Part model, mm, in its own coordinate system. Face numbers are marked on the shaded views. A direction names the side the tool comes from. Round coordinates to 2 decimals unless told otherwise and drop trailing zeros. Loops run counter-clockwise (first coordinate to the right, second up) from the corner with the lowest first, then second, coordinate; pieces in that order, holes last. Notation, with made-up numbers: M 32,30.25 L 79,30.25 A9 cw 79,42.25 Z; hole C -20,4.5 d7. An arc over 180 degrees is marked long. Answer as CSV lines item,"result". Start each with the question number.
Item 1: Drop flat-ended pins along their axis: pin 1 Ø4 at (x, y) = (-15.875, -15.875) entering from -Z; pin 2 Ø2.5 at (x, z) = (0.5, 1.5) entering from -Y; pin 3 Ø1 at (x, y) = (12.5, -40.5) entering from +Z. Give the stop position or say it passes through.
Item 2: Wall check: line 1 (Y direction, x = 0, z = 2.75); line 2 (Z direction, x = -20.25, y = -53); line 3 (Y direction, x = -7.5, z = 3.5). Give the ranges that are in metal, low to high.
Item 3: Band-saw the part on B-B (y = -53). Give the cut face in (x, z).
Item 4: Band-saw the part on D-D (z = 8.5). Give the cut face in (x, y), and give its area (3 significant figures).
Item 5: Band-saw the part on C-C (x = 0). Give the cut face in (y, z).
Item 6: Mould opens along X. For the marked faces 4, 5, 6 and 7 say: pulls with the +X half, pulls with the -X half, needs draft (parallel to the pull), parting line crosses it, or undercut.
Item 7: Which spindle directions (+Z, -Z, +X, -X, +Y, -Y) get a long thin tool onto all of the face, cutting with end or side? Do the marked faces 1, 2 and 3. Say none if no direction does.
Item 8: Band-saw the part on A-A (y = -30.5). Give the cut face in (x, z).
```python
from build123d import *

# Parameters (mm, degrees)
SKETCH_W        = 50
SKETCH_H        = 70
SKETCH_R        = 16
SKETCH_R_2      = 2.55
SKETCH_R_3      = 9.5
PAD_DEPTH       = 5
SKETCH001_W     = 12
SKETCH001_H     = 14
PAD001_DEPTH    = 10
SKETCH002_R     = 2.5
POCKET_DEPTH    = 25
SKETCH003_W     = 26
SKETCH003_H     = 4
POCKET001_DEPTH = 10
FILLET_R        = 4.99
FILLET001_R     = 2


with BuildPart() as part:
    # Sketch → Pad (new body)
    with BuildSketch(Plane.XY):
        with Locations((0, -11)):
            Rectangle(SKETCH_W, SKETCH_H)
        Circle(SKETCH_R, mode=Mode.SUBTRACT)
        with Locations((15.875, 15.875)):
            Circle(SKETCH_R_2, mode=Mode.SUBTRACT)
        with Locations((-15.875, 15.875)):
            Circle(SKETCH_R_2, mode=Mode.SUBTRACT)
        with Locations((-15.875, -15.875)):
            Circle(SKETCH_R_2, mode=Mode.SUBTRACT)
        with Locations((15.875, -15.875)):
            Circle(SKETCH_R_2, mode=Mode.SUBTRACT)
        with Locations((0, -30.5)):
            Circle(SKETCH_R_3, mode=Mode.SUBTRACT)
    extrude(amount=PAD_DEPTH)

    # Sketch001 → Pad001 (join)
    with BuildSketch(Plane.XY):
        with Locations((-19, -53)):
            Rectangle(SKETCH001_W, SKETCH001_H)
        with Locations((19, -53)):
            Rectangle(SKETCH001_W, SKETCH001_H)
    extrude(amount=PAD001_DEPTH)

    # Sketch002 → Pocket (cut, symmetric)
    with BuildSketch(Plane.YZ):
        with Locations((-53, 5)):
            Circle(SKETCH002_R)
    extrude(amount=POCKET_DEPTH, both=True, mode=Mode.SUBTRACT)

    # Sketch003 → Pocket001 (cut)
    with BuildSketch(Plane.XY):
        with Locations((0, -47)):
            Rectangle(SKETCH003_W, SKETCH003_H)
    extrude(amount=POCKET001_DEPTH, mode=Mode.SUBTRACT)

    # Fillet
    fillet_edges = [part.edges().sort_by_distance(p)[0] for p in [
        (-19, -46, 10),
        (-19, -60, 10),
        (-19, -60, 0),
        (19, -60, 0),
        (19, -60, 10),
        (19, -46, 10),
    ]]
    fillet(fillet_edges, radius=FILLET_R)

    # Fillet001
    fillet001_edges = [part.edges().sort_by_distance(p)[0] for p in [
        (25, 24, 2.5),
        (-25, 24, 2.5),
    ]]
    fillet(fillet001_edges, radius=FILLET001_R)


solid = part.part
```
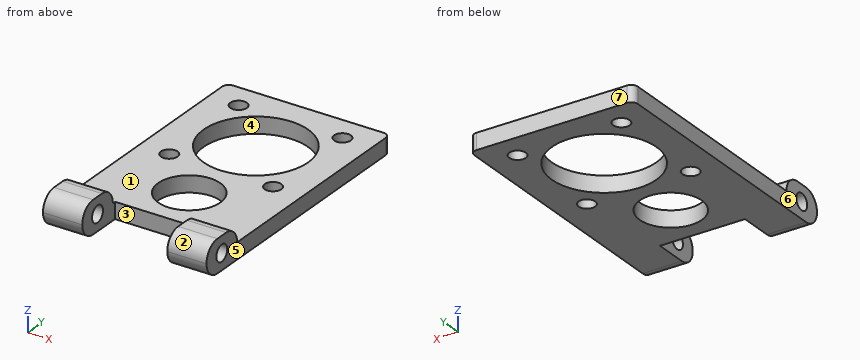
Answer block:
1,pin 1,"passes through"
1,pin 2,"stops at y = -45"
1,pin 3,"stops at z = 5"
2,line 1,"y = -45 to -40, -21 to -16, 16 to 24"
2,line 2,"z = 0 to 2.5, 7.5 to 10"
2,line 3,"y = -45 to -36.33, -24.67 to -14.13, 14.13 to 24"
3,outline,"M -25,0 L -13,0 L -13,2.5 L -25,2.5 Z; M -25,7.5 L -13,7.5 L -13,10 L -25,10 Z; M 13,0 L 25,0 L 25,2.5 L 13,2.5 Z; M 13,7.5 L 25,7.5 L 25,10 L 13,10 Z"
4,outline,"M -25,-58.58 L -13,-58.58 L -13,-47.42 L -25,-47.42 Z; M 13,-58.58 L 25,-58.58 L 25,-47.42 L 13,-47.42 Z"
4,area,"268 mm^2"
5,outline,"M -45,0 L -40,0 L -40,5 L -45,5 Z; M -21,0 L -16,0 L -16,5 L -21,5 Z; M 16,0 L 24,0 L 24,5 L 16,5 Z"
6,face 4,"undercut"
6,face 5,"pulls with the +X half"
6,face 6,"pulls with the -X half"
6,face 7,"needs draft"
7,face 1,"+Z, +X, -X, +Y"
7,face 2,"+Z, +X, -X, -Y"
7,face 3,"+Z, -Z, -Y"
8,outline,"M -25,0 L -9.5,0 L -9.5,5 L -25,5 Z; M 9.5,0 L 25,0 L 25,5 L 9.5,5 Z"
